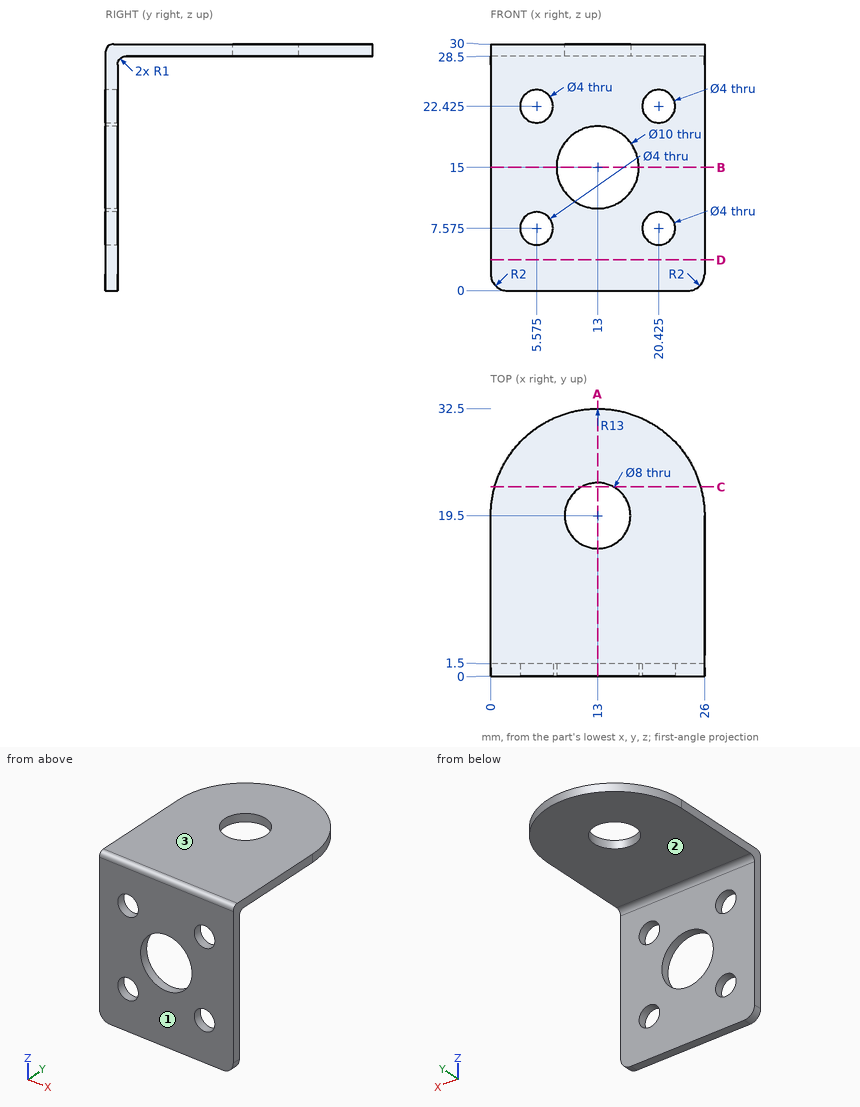
Study the drawing (mm; zero at the part's minimum x, y, z) and answer. Round coordinates to 2 decimals unless told otherwise and drop trailing zeros. Write each loop counter-clockwise with the first axis right and the second up, starting at its lowest first coordinate (ties: lowest second). Pieces come first, ordered by that corner, then holes. Notation, with made-up numbers: (40, 50.5) - (76, 50.5) arc R20 ccw to (76, 76.5) - close; hole circle Ø8 at (39, -24.75). An arc over 180 degrees is marked (long way). Return JSON: item names as keys, results as strings. Group by question number.
Q1. The part is cut by section D-D on z = 3.75. Write down the section's boundary in (x, y).
Q2. Each of these flat-tipped pins is pushed along its axis until it touches: pin 1 Ø8 at (x, z) = (10, 18.5) entering from +Y; pin 2 Ø2 at (x, y) = (17, 4.5) entering from -Z. Where does it stop, or does it pass through?
Q3. The part is cut by section A-A on x = 13. Write down the section's boundary in (y, z).
Q4. The part is cut by section B-B on z = 15. Write down the section's boundary in (x, y).
Q5. The part is cut by section C-C on y = 23. Write down the section's boundary in (x, z).
Q6. Find the intervals of material crossed by L1, parallel to X at y = 1.05, z = 15; L2, parallel to Y at x = 12.75, z = 25.75; L3, parallel to Z at x = 19.5, y = 26, in increasing order.
Q7. The mould has two halves that part along Z. Classify the marked faces 1, 2 and 3: released by +Z, released by -Z, zero draft, split by the parting line, or undercut.
Solved:
{
 "1": {"outline": "(0, 0) - (26, 0) - (26, 1.5) - (0, 1.5) - close"},
 "2": {"pin 1": "y = 1.5", "pin 2": "z = 28.5"},
 "3": {"outline": "(0, 0) - (1.5, 0) - (1.5, 10) - (0, 10) - close; (0, 20) - (1.5, 20) - (1.5, 27.5) arc R1 cw to (2.5, 28.5) - (15.5, 28.5) - (15.5, 30) - (1, 30) arc R1 ccw to (0, 29) - close; (23.5, 28.5) - (32.5, 28.5) - (32.5, 30) - (23.5, 30) - close"},
 "4": {"outline": "(0, 0) - (8, 0) - (8, 1.5) - (0, 1.5) - close; (18, 0) - (26, 0) - (26, 1.5) - (18, 1.5) - close"},
 "5": {"outline": "(0.48, 28.5) - (11.06, 28.5) - (11.06, 30) - (0.48, 30) - close; (14.94, 28.5) - (25.52, 28.5) - (25.52, 30) - (14.94, 30) - close"},
 "6": {"L1": "0 to 8, 18 to 26", "L2": "0 to 1.5", "L3": "28.5 to 30"},
 "7": {"face 1": "zero draft", "face 2": "released by -Z", "face 3": "released by +Z"}
}
